Verification items for the finished model (mm, model axes). Face numbers are marked on the shaded views. A direction names the side the tool comes from. Give positions to 0.01 mm unless a question says otherwise; leave off trailing zeros. Loops run counter-clockwise (first coordinate to the right, second up) from the corner with the lowest first, then second, coordinate; pieces in that order, holes last. Notation, with made-up numbers: M 13.5,35 L 63.5,35 A10 ccw 63.5,54 Z; hole C 63,66 d1. An arc over 180 degrees is marked long. Use CSV: the item, a comma, the result in double quotes.
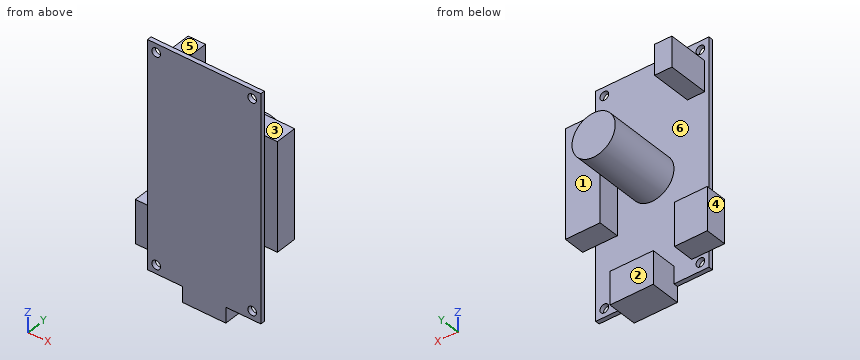
Autodesk Fusion 360 part; units mm, degrees
sketch "Sketch1" plane through (0, 0, 0) normal (0, 1, 0) x (1, 0, 0)
  line L0 (0, 0) -> (26.2, 0)
  line L1 (26.2, 0) -> (26.2, -52)
  line L2 (26.2, -52) -> (0, -52)
  line L3 (0, -52) -> (0, 0)
  circle A0 centre (2, -2) radius 1
  circle A1 centre (24.2, -2) radius 1
  line L4 (0, -26) -> (26.2, -26)
  circle A2 centre (2, -50) radius 1
  circle A3 centre (24.2, -50) radius 1
  dimension "d1" = 52
  dimension "d2" = 26.2
  dimension "d3" = 2
  dimension "d4" = 2
  dimension "d5" = 2
  dimension "d6" = 2
  dimension "d7" = 2
  dimension "d8" = 2
extrude "Extrude1" add sketch "Sketch1" along normal blind 1
sketch "Sketch2" plane through (0, 1, 0) normal (0, 1, 0) x (-1, 0, 0)
  circle A0 centre (-2, 2) radius 1
  circle A1 centre (-24.2, 2) radius 1
  circle A2 centre (-2, 50) radius 1
  circle A3 centre (-24.2, 50) radius 1
  line L0 (0, 52) -> (-26.2, 52)
  line L1 (-26.2, 52) -> (-26.2, 0)
  line L2 (-26.2, 0) -> (0, 0)
  line L3 (0, 0) -> (0, 52)
  line L4 (-1, 47.0961) -> (-5, 47.0961)
  line L5 (-5, 47.0961) -> (-5, 40.0961)
  line L6 (-5, 40.0961) -> (-1, 40.0961)
  line L7 (-1, 40.0961) -> (-1, 47.0961)
  line L8 (-21.2, 42) -> (-29.2, 42)
  line L9 (-29.2, 42) -> (-29.2, 17)
  line L10 (-29.2, 17) -> (-21.2, 17)
  line L11 (-21.2, 17) -> (-21.2, 42)
  line L12 (0, 3.6) -> (-4, 3.6)
  line L13 (-4, 3.6) -> (-4, 13.6)
  line L14 (-4, 13.6) -> (0, 13.6)
  line L15 (0, 13.6) -> (0, 3.6)
  line L16 (0, 3.6) -> (3.6, 3.6)
  line L17 (3.6, 3.6) -> (3.6, 13.6)
  line L18 (3.6, 13.6) -> (0, 13.6)
  line L19 (0, 13.6) -> (0, 3.6)
  dimension "d11" = 4
  dimension "d12" = 7
  dimension "d15" = 3
  dimension "d16" = 25
  dimension "d17" = 8
  dimension "d18" = 10
  dimension "d29" = 4
  dimension "d30" = 10
  dimension "d31" = 3.6
  dimension "d32" = 3.6
extrude "Extrude2" add sketch "Sketch2" along normal blind 9.5 contours L4 L5 L6 L7
extrude "Extrude3" add sketch "Sketch2" along normal blind 5 contours L1 L8 L10 L11 | L1 L8 L9 L10
sketch "Sketch3" plane through (0, 0, 0) normal (0, -1, 0) x (1, 0, 0)
  circle A0 centre (2, 2) radius 1
  circle A1 centre (24.2, 2) radius 1
  circle A2 centre (2, 50) radius 1
  circle A3 centre (24.2, 50) radius 1
  line L0 (26.2, 52) -> (0, 52)
  line L1 (0, 52) -> (0, 0)
  line L2 (0, 0) -> (26.2, 0)
  line L3 (26.2, 0) -> (26.2, 52)
  circle A4 centre (13.1, 26) radius 5
  line L4 (18.1, 0) -> (8.1, 0)
  line L5 (8.1, 0) -> (8.1, 4)
  line L6 (8.1, 4) -> (18.1, 4)
  line L7 (18.1, 4) -> (18.1, 0)
  line L8 (8.1, 0) -> (0, 0)
  line L9 (18.1, 0) -> (26.2, 0)
  line L10 (8.1, 0) -> (18.1, 0)
  line L11 (18.1, 0) -> (18.1, -3.6)
  line L12 (18.1, -3.6) -> (8.1, -3.6)
  line L13 (8.1, -3.6) -> (8.1, 0)
  point P0 (13.1, 26)
  dimension "d21" = 10
  dimension "d24" = 10
  dimension "d25" = 4
  dimension "d26" = 3.6
extrude "Extrude4" add sketch "Sketch3" against normal blind 18 contours A4
extrude "Extrude5" add sketch "Sketch3" against normal blind 7 contours L2 L4 L10 L11 L12 L13 | L2 L4 L5 L6 L7 L10
extrude "Extrude6" add sketch "Sketch2" along normal blind 5 contours L3 L15 L16 L17 L18 L19 | L3 L12 L13 L14 L15 L19
(1) Section check B-B on x = 24.2. Record the cut outline in (y, z), plus the area to 3 significant figures.
Calculated:
outline,"M 0,0 L 1,0 L 1,1 L 0,1 Z; M 0,3 L 1,3 L 1,17 L 6,17 L 6,42 L 1,42 L 1,49 L 0,49 Z; M 0,51 L 1,51 L 1,52 L 0,52 Z"
area,"173 mm²"
(2) Mould release check, pull along Z, two halves, no side actions. Record for the marked faces 4, 5 and 6: released by +Z, released by -Z, zero draft, split by the parting line, or undercut.
Calculated:
face 4,"zero draft"
face 5,"released by +Z"
face 6,"undercut"
(3) Scan lines: L1, parallel to Z at x = 24.2, y = 0.6; L2, parallel to X at y = 0.3, z = 50; L3, parallel to Y at x = 10, z = 11. Record each from-to range of solid material in increasing order. Write a range as from..to.
Calculated:
L1,"z = 0..1, 3..49, 51..52"
L2,"x = 0..1, 3..23.2, 25.2..26.2"
L3,"y = 0..1"
(4) Section check D-D on y = 3.5. Record the cut outline in (x, z), plus the area to 3 significant figures.
Calculated:
outline,"M -3.6,3.6 L 4,3.6 L 4,13.6 L -3.6,13.6 Z; M 1,40.1 L 5,40.1 L 5,47.1 L 1,47.1 Z; M 8.1,-3.6 L 18.1,-3.6 L 18.1,4 L 8.1,4 Z; C 13.1,26 d10; M 21.2,17 L 29.2,17 L 29.2,42 L 21.2,42 Z"
area,"459 mm²"
(5) Section check C-C on y = 7.75. Record the cut outline in (x, z).
Calculated:
outline,"M 1,40.1 L 5,40.1 L 5,47.1 L 1,47.1 Z; C 13.1,26 d10"
(6) Depth check by flat-ended pin: pin 1 Ø0.8 at (x, y) = (23, 0.5) entering from -Z; pin 2 Ø1.5 at (y, z) = (2.5, 31) entering from -X; pin 3 Ø5 at (y, z) = (10.5, 2) entering from -X; pin 4 Ø6.5 at (x, z) = (23.5, 34.5) entering from +Y. Enter the tip coordinate at first touch or a pass-through.
Calculated:
pin 1,"stops at z = 0"
pin 2,"stops at x = 10.47"
pin 3,"passes through"
pin 4,"stops at y = 6"
(7) Tool access check on the marked faces 1, 2 and 3. Record the directions out of +Z, -Z, +X, -X, +Y, -Y that give a thin tool (end or side, any length) a straight path to the whole face; none if there is none.
Calculated:
face 1,"+Z, -Z, +X, +Y"
face 2,"-Z, +X, -X, +Y"
face 3,"+Z, +X, +Y"
(8) Section check A-A on z = 2. Record the cut outline in (x, y), plus the area to 3 significant figures.
Calculated:
outline,"M 0,0 L 1,0 L 1,1 L 0,1 Z; M 3,0 L 23.2,0 L 23.2,1 L 18.1,1 L 18.1,7 L 8.1,7 L 8.1,1 L 3,1 Z; M 25.2,0 L 26.2,0 L 26.2,1 L 25.2,1 Z"
area,"82.2 mm²"
